```python
from build123d import *

# Parameters (mm, degrees)
SKETCH1_R                          = 12.446
EXTRUDE1_DEPTH                     = 6.0071
CHAMFER1_SIZE                      = 1.524
SKETCH2_R                          = 11.5951
EXTRUDE2_DEPTH                     = 0.99076
SKETCH3_R                          = 1.5875
EXTRUDE3_DEPTH                     = 6.3754
F_5_16_0_3125_DIAMETER_HOLE2_D     = 5.1562
F_5_16_0_3125_DIAMETER_HOLE2_DEPTH = 0.381
M3X0_5_TAPPED_HOLE1_D              = 2.5
M3X0_5_TAPPED_HOLE1_DEPTH          = 5.3086
M3X0_5_TAPPED_HOLE1_TIP            = 0.751075774


with BuildPart() as part:
    # Sketch1 → Extrude1 (new body, symmetric)
    with BuildSketch(Plane(origin=(0, 0, 0), x_dir=(1, 0, 0), z_dir=(0, 1, 0))):
        with Locations(Location((0, 0, 0), (0, 0, 270))):  # turned: the seam where the file's is
            Circle(SKETCH1_R)
    extrude(amount=EXTRUDE1_DEPTH, both=True)

    # Chamfer1
    chamfer1_edges = [part.edges().sort_by_distance(p)[0] for p in [
        (0, 6.0071, -12.446),
    ]]
    chamfer(chamfer1_edges, length=CHAMFER1_SIZE)

    # Sketch2 → Extrude2 (add)
    with BuildSketch(Plane.XZ.offset(6.0071)):
        with Locations(Location((0, 0, 0), (0, 0, 90))):  # turned: the seam where the file's is
            Circle(SKETCH2_R)
    extrude(amount=EXTRUDE2_DEPTH)

    # Sketch3 → Extrude3 (cut)
    with BuildSketch(Plane(origin=(0, 6.0071, 0), x_dir=(1, 0, 0), z_dir=(0, 1, 0))):
        with Locations(Location((0, 0, 0), (0, 0, 270))):  # turned: the seam where the file's is
            Circle(SKETCH3_R)
    extrude(amount=-EXTRUDE3_DEPTH, mode=Mode.SUBTRACT)

    # Sketch4 → Cut-Revolve1 (revolve, cut)
    with BuildSketch(Plane.XY):
        with BuildLine():
            Line((0, 13.035099954), (0, -0.004899954))
            ThreePointArc((0, -0.004899954), (6.519999954, 6.5151), (0, 13.035099954))
        make_face()
    revolve(axis=Axis((0, 13.035099954, 0), (0, -1, 0)), mode=Mode.SUBTRACT)

    # 5/16 (0.3125) Diameter Hole2
    with Locations(Plane(origin=(12.446, 0, 0), x_dir=(0, 0, -1), z_dir=(1, 0, 0))):
        with Locations((0, -0.6223)):
            Hole(F_5_16_0_3125_DIAMETER_HOLE2_D / 2, depth=F_5_16_0_3125_DIAMETER_HOLE2_DEPTH)

    # M3x0.5 Tapped Hole1
    with Locations(Plane(origin=(12.065, 0, 0), x_dir=(0, 0, -1), z_dir=(1, 0, 0))):
        with Locations((0, -0.6223)):
            Hole(M3X0_5_TAPPED_HOLE1_D / 2, depth=M3X0_5_TAPPED_HOLE1_DEPTH)
            with Locations((0, 0, -(M3X0_5_TAPPED_HOLE1_DEPTH + M3X0_5_TAPPED_HOLE1_TIP / 2))):  # 118° drill point
                Cone(0, M3X0_5_TAPPED_HOLE1_D / 2, M3X0_5_TAPPED_HOLE1_TIP, mode=Mode.SUBTRACT)


solid = part.part
```
Here's how the part is built. I have some questions about the finished solid (model axes, mm). A direction names the side the tool comes from. Coordinates: 2 decimals unless noted, no trailing zeros. Loops run counter-clockwise (first coordinate to the right, second up) from the corner with the lowest first, then second, coordinate; pieces in that order, holes last. Notation, with made-up numbers: (38, 34) - (43, 34) arc R12 ccw to (43, 57) - close; hole circle Ø4 at (61.25, 29.25). An arc over 180 degrees is marked (long way). Return JSON: item names as keys, results as strings. Group by question number.
Item 1: Will these pins go through, and if not, where does the flat tip stop? P1, Ø1, axis at x = -0.5, z = 0, coming from the +Y side; P2, Ø3, axis at y = 1.5, z = -6, coming from the +X side; P3, Ø3, axis at x = 5.5, y = -3, coming from the -Z side.
Item 2: If we section it at A-A on x = 0: Write out the boundary of the cut face in (y, z), and give its area (3 significant figures).
Item 3: If we section it at B-B on y = 3: Write out the boundary of the cut face in (x, z), and give its area (3 significant figures).
Item 4: I need wall thicknesses on line 1 (Y direction, x = 10, z = 0); line 2 (X direction, y = 2.5, z = -4); line 3 (Y direction, x = 12.3, z = 0). Which ranges of each line are inside material? Lowest first, please. Write a range as from..to.
Item 5: We'd pull the mould along X, two halves only. Please class faces 1 (the face through (9.374, -1.383, -0.992)), 2 (the face through (0, -0.368, 0)), 3 (the face through (-4.2, 5.9, 10.2)): +X half, -X half, draft (parallel to the pull), parting line (faces both ways), or undercut.
Item 6: On a 3-axis mill with a long thin cutter (end or side, diameter ignored), from which of +Z, -Z, +X, -X, +Y, -Y can I reach the whole of each face in a straight line? I mean faces 4 (the face through (-5, 6.007, 5)), 5 (the face through (-0.966, -0.085, -1.26)), 6 (the face through (12.065, -2, -1)), 7 (the face through (11.32, -6.5, -2.51)), 8 (the face through (-11.042, -0.689, 5.743)). Say none if no direction works.
Calculated:
{
 "1": {"P1": "stops at y = -0.37", "P2": "stops at x = 11.6", "P3": "stops at z = -11.79"},
 "2": {"outline": "(-7, -11.6) - (-6.01, -11.6) - (-6.01, -12.45) - (4.48, -12.45) - (6.01, -10.92) - (6.01, -6.5) arc R6.52 cw to (0.19, -1.59) - (-0.37, -1.59) - (-0.37, 1.59) - (0.19, 1.59) arc R6.52 cw to (6.01, 6.5) - (6.01, 10.92) - (4.48, 12.45) - (-6.01, 12.45) - (-6.01, 11.6) - (-7, 11.6) - close", "area": "258 mm^2"},
 "3": {"outline": "circle Ø24.89 at (0, 0); hole circle Ø10.98 at (0, 0)", "area": "392 mm^2"},
 "4": {"line 1": "y = -7..-1.87, 0.63..6.01", "line 2": "x = -11.79..-3.22, 3.22..11.79", "line 3": "y = -6.01..-3.2, 1.96..4.63"},
 "5": {"face 1": "draft", "face 2": "undercut", "face 3": "parting line"},
 "6": {"face 4": "+Z, -Z, +X, -X, +Y", "face 5": "+Y", "face 6": "+X", "face 7": "-Y", "face 8": "+Y, -Y"}
}
